The model under review builds one solid part; all positions refer to its coordinate system, in mm. Round coordinates to 2 decimals unless told otherwise and drop trailing zeros. Write each loop counter-clockwise with the first axis right and the second up, starting at its lowest first coordinate (ties: lowest second). Pieces come first, ordered by that corner, then holes. Notation, with made-up numbers: (37.25, 2) -> (94.25, 2) arc R19 ccw to (94.25, 16) -> close; hole circle Ø5 at (-4.5, -17). An arc over 180 degrees is marked (long way). Return JSON: item names as keys, results as strings. Group by question number.
1. For line 1 along Y through (x, z) = (0, 20.25); line 2 along Z through (x, y) = (-100, -131.5); line 3 along X through (y, z) = (-45, 68.5), list the stretches that pass through material, from the lowest coordinate up. Write a range as from..to.
2. Clearance check with flat-ended pins moving along their axes: P1, Ø3, axis at y = -62.5, z = 34.5, coming from the -X side; P2, Ø8, axis at y = -52, z = 36.5, coming from the -X side; P3, Ø3, axis at y = 69, z = 68, coming from the +X side. State where each tip first meets the part, or that it passes through.
3. Take a section at A-A, the plane z = 56. Write out the cut boundary in (x, y), then the cut area to 3 significant figures.
from build123d import *

# Parameters (mm, degrees)
F2_R     = 6.35
F4_D     = 50.8
F4_DEPTH = 50.8
F4_TIP   = 15.2618597233


with BuildPart() as f1:
    # F0 (on Front) → F1 (revolve)
    with BuildSketch(Plane.XZ):
        Polygon((0, 12.7), (0, 0), (304.8, 0), (304.8, 25.4), (50.8, 152.4), (0, 152.4), (0, 76.2), (50.8, 76.2), (50.8, 138.2009683429), (279.4, 23.9009683429), (279.4, 12.7), align=None)
    revolve(axis=Axis((0, 0, 114.3), (0, 0, 1)))

    # F2
    f2_edges = [f1.edges().sort_by_distance(p)[0] for p in [
        (-304.8, 0, 25.4),
    ]]
    fillet(f2_edges, radius=F2_R)

    # F4
    with Locations(Plane.XY.offset(152.4)):
        with Locations((0, 0)):
            Hole(F4_D / 2, depth=F4_DEPTH)
            with Locations((0, 0, -(F4_DEPTH + F4_TIP / 2))):  # 118° drill point
                Cone(0, F4_D / 2, F4_TIP, mode=Mode.SUBTRACT)


solid = f1.part
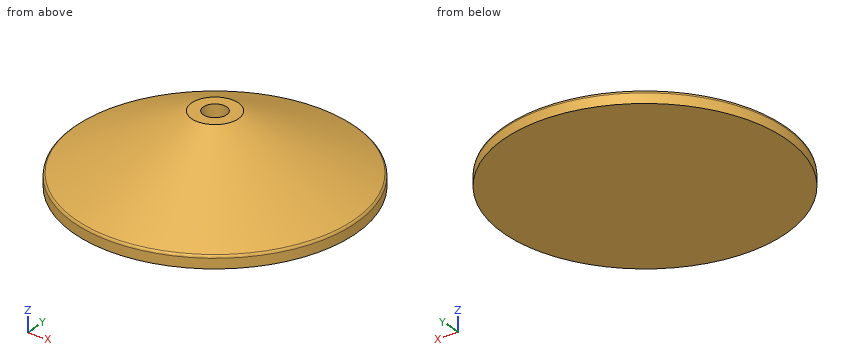
Output:
{
 "1": {"line 1": "y = -304.8..-279.4, 279.4..304.8", "line 2": "z = 0..12.7, 81..95.2", "line 3": "x = -213.92..-184.8, 184.8..213.92"},
 "2": {"P1": "stops at x = -282.79", "P2": "stops at x = -285.94", "P3": "stops at x = 211.67"},
 "3": {"outline": "circle Ø487.2 at (0, 0); hole circle Ø430.4 at (0, 0)", "area": "40,900 mm^2"}
}
